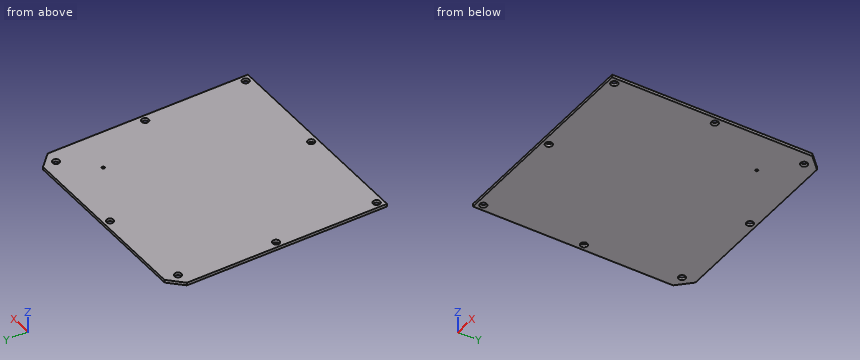
Autodesk Inventor part; units mm, degrees
ref_plane "YZ Plane" through (0, 0, 0) normal (1, 0, 0) x (0, 1, 0)
ref_plane "XZ Plane" through (0, 0, 0) normal (0, 1, 0) x (-1, 0, 0)
ref_plane "XY Plane" through (0, 0, 0) normal (0, 0, 1) x (1, 0, 0)
sketch "Sketch1" plane through (0, 0, 0) normal (0, 0, 1) x (1, 0, 0)
  line L0 (230, 0) -> (0, 0)
  line L1 (14.5, 230) -> (215.5, 230)
  line L2 (0, 215.5) -> (0, 0)
  line L3 (0, 215.5) -> (14.5, 230)
  line L4 (230, 215.5) -> (230, 0)
  line L5 (215.5, 230) -> (230, 215.5)
  dimension "d6" = 135
  dimension "d7" = 230
  dimension "d8" = 230
  dimension "d9" = 315.0161
  dimension "d10" = 152.3815
extrude "Extrusion1" add sketch "Sketch1" along normal blind 3
sketch "Sketch2" plane through (0, 0, 3) normal (0, 0, 1) x (1, 0, 0)
  line L0 (215.5, 230) -> (14.5, 230)
  circle A0 centre (115, 223.25) radius 3.75
  line L1 (0, 0) -> (230, 0)
  circle A1 centre (115, 6.75) radius 3.75
  line L2 (0, 215.5) -> (0, 0)
  circle A2 centre (6.75, 115) radius 3.75
  line L3 (230, 0) -> (230, 215.5)
  circle A3 centre (223.25, 115) radius 3.75
  circle A4 centre (6.75, 6.75) radius 3.75
  circle A5 centre (223.25, 6.75) radius 3.75
  line L4 (14.5, 230) -> (0, 215.5)
  circle A6 centre (14.1443, 215.8557) radius 3.75
  line L5 (230, 215.5) -> (215.5, 230)
  circle A7 centre (215.8557, 215.8557) radius 3.75
  circle A8 centre (185, 185) radius 1.5
  dimension "d19" = 7.5
  dimension "d21" = 7.5
  dimension "d23" = 7.5
  dimension "d25" = 7.5
  dimension "d28" = 7.5
  dimension "d31" = 7.5
  dimension "d34" = 7.5
  dimension "d37" = 7.5
  dimension "d43" = 3
extrude "Extrusion2" cut sketch "Sketch2" against normal through all contours A0 | A1 | A2 | A3 | A4 | A5 | A6 | A7 | A8
properties part number "tampa da caixa de engrenagem"
Could you check a few things on this model? Use its own coordinates, in mm. Coordinates: 2 decimals unless noted, no trailing zeros. Write each loop counter-clockwise with the first axis right and the second up, starting at its lowest first coordinate (ties: lowest second). Pieces come first, ordered by that corner, then holes. Notation, with made-up numbers: (6.25, 33) - (58.25, 33) arc R20 cw to (58.25, 62) - close; hole circle Ø2 at (72.5, -32). An arc over 180 degrees is marked (long way). Put each result on its own line as item: value. Start each with the question number.
Q1. I want a section at A-A on y = 6.75. Write out the boundary of the cut face in (x, z), plus the area to 4 significant figures.
Q2. I want a section at C-C on y = 223.25. Write out the boundary of the cut face in (x, z), plus the area to 3 significant figures.
Q3. I want a section at D-D on y = 115. Write out the boundary of the cut face in (x, z), plus the area to 3 significant figures.
Q4. Please list where these lines run through material, in increasing order: L1, parallel to Y at x = 115, z = 1; L2, parallel to Y at x = 6.75, z = 1.45; L3, parallel to Y at x = 185, z = 1.4.
Q5. I want a section at B-B on x = 6.75. Write out the boundary of the cut face in (y, z).
Checks:
1. outline: (0, 0) - (3, 0) - (3, 3) - (0, 3) - close; (10.5, 0) - (111.25, 0) - (111.25, 3) - (10.5, 3) - close; (118.75, 0) - (219.5, 0) - (219.5, 3) - (118.75, 3) - close; (227, 0) - (230, 0) - (230, 3) - (227, 3) - close
1. area: 622.5 mm²
2. outline: (7.75, 0) - (111.25, 0) - (111.25, 3) - (7.75, 3) - close; (118.75, 0) - (222.25, 0) - (222.25, 3) - (118.75, 3) - close
2. area: 621 mm²
3. outline: (0, 0) - (3, 0) - (3, 3) - (0, 3) - close; (10.5, 0) - (219.5, 0) - (219.5, 3) - (10.5, 3) - close; (227, 0) - (230, 0) - (230, 3) - (227, 3) - close
3. area: 645 mm²
4. L1: 0 to 3, 10.5 to 219.5, 227 to 230
4. L2: 0 to 3, 10.5 to 111.25, 118.75 to 222.25
4. L3: 0 to 183.5, 186.5 to 230
5. outline: (0, 0) - (3, 0) - (3, 3) - (0, 3) - close; (10.5, 0) - (111.25, 0) - (111.25, 3) - (10.5, 3) - close; (118.75, 0) - (222.25, 0) - (222.25, 3) - (118.75, 3) - close
